Geometry: final body of the model. Coordinates: model frame, mm. A direction names the side the tool comes from. Round coordinates to 2 decimals unless told otherwise and drop trailing zeros. Loops run counter-clockwise (first coordinate to the right, second up) from the corner with the lowest first, then second, coordinate; pieces in that order, holes last. Notation, with made-up numbers: (16, 33.5) - (69, 33.5) arc R27 cw to (69, 72.5) - close; hole circle Ø7 at (-35.75, 41.25). An arc over 180 degrees is marked (long way). Use CSV: the item, a comma, the result in double quotes.
from build123d import *

# Parameters (mm, degrees)
BOSS_EXTRUDE1_DEPTH = 168
BOSS_EXTRUDE2_DEPTH = 2


with BuildPart() as part:
    # Sketch1 → Boss-Extrude1 (new body)
    with BuildSketch(Plane(origin=(0, 0, 0), x_dir=(1, 0, 0), z_dir=(0, 1, 0))):
        with BuildLine():
            Line((0, 205), (0, 200))
            ThreePointArc((0, 200), (200, 0), (0, -200))
            Line((0, -200), (0, -205))
            ThreePointArc((0, -205), (205, 0), (0, 205))
        make_face()
    extrude(amount=BOSS_EXTRUDE1_DEPTH)

    # Sketch2 → Boss-Extrude2 (add)
    with BuildSketch(Plane(origin=(0, 0, 0), x_dir=(1, 0, 0), z_dir=(0, 1, 0))):
        with BuildLine():
            Line((87.177978871, -180), (74.10128204, -153))
            ThreePointArc((74.10128204, -153), (136.845155159, -100.863291189), (168.076619433, -25.5))
            Line((168.076619433, -25.5), (197.737199333, -30))
            ThreePointArc((197.737199333, -30), (160.994300187, -118.662695517), (87.177978871, -180))
        make_face()
        with BuildLine():
            Line((197.737199333, 30), (168.076619433, 25.5))
            ThreePointArc((168.076619433, 25.5), (136.845155159, 100.863291189), (74.10128204, 153))
            Line((74.10128204, 153), (87.177978871, 180))
            ThreePointArc((87.177978871, 180), (160.994300187, 118.662695517), (197.737199333, 30))
        make_face()
    boss_extrude2 = extrude(amount=BOSS_EXTRUDE2_DEPTH)

    # Mirror2: Boss-Extrude2 across plane
    add(boss_extrude2.mirror(Plane.ZX.offset(84)))


solid = part.part
Item 1: Mould query, pull axis Y, two halves, no side actions, for faces 1 (the cylindrical face through (199.95, 82.82, -4.4)), 2 (the cylindrical face through (136, 1, 102)), 3 (the flat face through (170, 0, 29)), 4 (the flat face through (170, 168, 29)). Classes: released by +Y, released by -Y, zero draft, split by the parting line, or undercut.
Final values:
face 1,"undercut"
face 2,"zero draft"
face 3,"released by -Y"
face 4,"released by +Y"
Item 2: Section D-D on y = 93. Return the cut outline in (x, z), plus the area to 3 significant figures.
Final values:
outline,"(0, -205) arc R205 ccw to (0, 205) - (0, 200) arc R200 cw to (0, -200) - close"
area,"3,180 mm²"
Item 3: Section C-C on z = 83.5. Return the cut outline in (x, y), plus the area to 3 significant figures.
Final values:
outline,"(148.08, 0) - (187.22, 0) - (187.22, 168) - (148.08, 168) - (148.08, 166) - (181.74, 166) - (181.74, 2) - (148.08, 2) - close"
area,"1,060 mm²"
Item 4: Section B-B on x = 79. Return the cut outline in (y, z), plus the area to 3 significant figures.
Final values:
outline,"(0, -189.17) - (168, -189.17) - (168, -183.74) - (0, -183.74) - close; (0, -163.11) - (2, -163.11) - (2, -150.53) - (0, -150.53) - close; (0, 150.53) - (2, 150.53) - (2, 163.11) - (0, 163.11) - close; (0, 183.74) - (168, 183.74) - (168, 189.17) - (0, 189.17) - close; (166, -163.11) - (168, -163.11) - (168, -150.53) - (166, -150.53) - close; (166, 150.53) - (168, 150.53) - (168, 163.11) - (166, 163.11) - close"
area,"1,930 mm²"
Item 5: Reachability of faces 5 (the flat face through (80.73, 167.01, 166.69)), 6 (the flat face through (145, 2, 102)), 7 (the cylindrical face through (204.95, 82.82, 4.51)) from +Z, -Z, +X, -X, +Y, -Y: full face, straight path, thin tool, end or side. Return the list, or none.
Final values:
face 5,"-X, +Y, -Y"
face 6,"-X"
face 7,"+X, +Y, -Y"
Item 6: Section A-A on x = 43. Return the cut outline in (y, z), plus the area to 3 significant figures.
Final values:
outline,"(0, -200.44) - (168, -200.44) - (168, -195.32) - (0, -195.32) - close; (0, 195.32) - (168, 195.32) - (168, 200.44) - (0, 200.44) - close"
area,"1,720 mm²"
Item 7: Pin query (flat end, axial travel): P1, Ø3, axis at y = 66.5, z = -102.5, coming from the -X side; P2, Ø10, axis at y = 108.5, z = 109, coming from the +X side; P3, Ø1.5, axis at y = 91.5, z = -20.5, coming from the +X side. Return the tip coordinate at first contact, or that it passes through.
Final values:
P1,"stops at x = 170.83"
P2,"stops at x = 176.66"
P3,"stops at x = 204.05"
Item 8: Material intervals for line 1 (Y direction, x = 181, z = -52); line 2 (Z direction, x = 44.5, y = 157.5); line 3 (Z direction, x = 154, y = 117), sorted ascending.
Final values:
line 1,"y = 0 to 2, 166 to 168"
line 2,"z = -200.11 to -194.99, 194.99 to 200.11"
line 3,"z = -135.31 to -127.61, 127.61 to 135.31"
